```python
from build123d import *

# Parameters (mm, degrees)
PAD_DEPTH       = 15
PAD_DEPTH_BACK  = 15
SKETCH001_R     = 1.6
HOLE_DEPTH      = 25
SKETCH002_R     = 1.1
POCKET_DEPTH    = 5.801
SKETCH003_R     = 4.75
POCKET001_DEPTH = 5


with BuildPart() as part:
    # Sketch → Pad (new body, two sides)
    with BuildSketch(Plane.YZ) as pad_sk:
        Polygon((-21, 0), (-21, -5.8), (-16.2, -5.8), (-16.2, -3.3), (-15.2, -3.3), (-15.2, -1.8), (15.2, -1.8), (15.2, -3.3), (16.2, -3.3), (16.2, -5.8), (21, -5.8), (21, 0), align=None)
    extrude(amount=PAD_DEPTH)
    extrude(pad_sk.sketch, amount=-PAD_DEPTH_BACK)

    # Sketch001 → Hole (cut)
    with BuildSketch(Plane.XY):
        with Locations((-10, 17.5)):
            Circle(SKETCH001_R)
        with Locations((0, 17.5)):
            Circle(SKETCH001_R)
        with Locations((10, 17.5)):
            Circle(SKETCH001_R)
        with Locations((10, -17.5)):
            Circle(SKETCH001_R)
        with Locations((0, -17.5)):
            Circle(SKETCH001_R)
        with Locations((-10, -17.5)):
            Circle(SKETCH001_R)
    extrude(amount=-HOLE_DEPTH, mode=Mode.SUBTRACT)

    # Sketch002 → Pocket (cut, through all)
    with BuildSketch(Plane.XY):
        with Locations((-10, 10)):
            Circle(SKETCH002_R)
        with Locations((10, 10)):
            Circle(SKETCH002_R)
        with Locations((10, -10)):
            Circle(SKETCH002_R)
        with Locations((-10, -10)):
            Circle(SKETCH002_R)
    extrude(amount=-POCKET_DEPTH, mode=Mode.SUBTRACT)

    # Sketch003 → Pocket001 (cut)
    with BuildSketch(Plane.XY):
        with Locations((-8, 0)):
            Circle(SKETCH003_R)
        with Locations((8, 0)):
            Circle(SKETCH003_R)
    extrude(amount=-POCKET001_DEPTH, mode=Mode.SUBTRACT)


solid = part.part
```
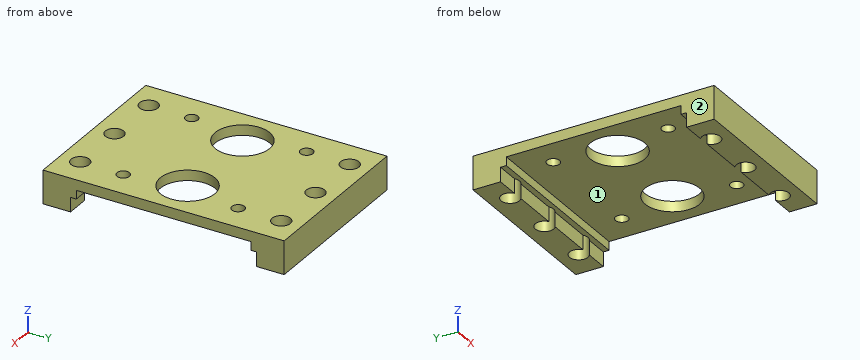
The model under review builds one solid part; all positions refer to its coordinate system, in mm. Face numbers are marked on the shaded views. A direction names the side the tool comes from. Round coordinates to 2 decimals unless told otherwise and drop trailing zeros. Write each loop counter-clockwise with the first axis right and the second up, starting at its lowest first coordinate (ties: lowest second). Pieces come first, ordered by that corner, then holes.
(1) Machinability: for the marked faces 1 and 2, which of the approach directions +Z, -Z, +X, -X, +Y, -Y give a long, thin tool a straight path to every point of the face, cutting with its end or side? Answer none if there is none.
(2) We need section B-B on y = 2.5. Give the boundary of the cut face in (x, z), and give its area (3 significant figures).
(3) We need section A-A on z = -4.25. Give the boundary of the cut face in (x, y).
(4) Insertion check: pin 1 (1 mm diameter, centred on x = -5, y = -11, fed in from -Z). The pin has a flat end and moves straight along its axis. Give the tip position at first contact, or say it passes through.
(5) We need section D-D on x = -5.5. Give the boundary of the cut face in (y, z), and give its area (3 significant figures).
(6) Wall thickness on L1, parallel to X at y = -17.5, z = -1.5; L2, parallel to Y at x = -10, z = -2.75; L3, parallel to Y at x = 0, z = -1.5: over which ranges is each line inside the solid? List them lowest first.
(7) We need section C-C on x = 10. Give the boundary of the cut face in (y, z), and give its area (3 significant figures).
Findings below:
1. face 1: -Z, +X, -X
1. face 2: +Z, -Z, -X, +Y, -Y
2. outline: (-15, -1.8) - (-12.04, -1.8) - (-12.04, 0) - (-15, 0) - close; (-3.96, -1.8) - (3.96, -1.8) - (3.96, 0) - (-3.96, 0) - close; (12.04, -1.8) - (15, -1.8) - (15, 0) - (12.04, 0) - close
2. area: 24.9 mm2
3. outline: (-15, -21) - (15, -21) - (15, -16.2) - (10.93, -16.2) arc R1.6 cw (long way) to (9.07, -16.2) - (0.93, -16.2) arc R1.6 cw (long way) to (-0.93, -16.2) - (-9.07, -16.2) arc R1.6 cw (long way) to (-10.93, -16.2) - (-15, -16.2) - close; (-15, 16.2) - (-10.93, 16.2) arc R1.6 cw (long way) to (-9.07, 16.2) - (-0.93, 16.2) arc R1.6 cw (long way) to (0.93, 16.2) - (9.07, 16.2) arc R1.6 cw (long way) to (10.93, 16.2) - (15, 16.2) - (15, 21) - (-15, 21) - close
4. pin 1: stops at z = -1.8
5. outline: (-21, -5.8) - (-16.2, -5.8) - (-16.2, -3.3) - (-15.2, -3.3) - (-15.2, -1.8) - (-4.04, -1.8) - (-4.04, 0) - (-21, 0) - close; (4.04, -1.8) - (15.2, -1.8) - (15.2, -3.3) - (16.2, -3.3) - (16.2, -5.8) - (21, -5.8) - (21, 0) - (4.04, 0) - close
5. area: 102 mm2
6. L1: x = -15 to -11.6, -8.4 to -1.6, 1.6 to 8.4, 11.6 to 15
6. L2: y = -21 to -19.1, -15.9 to -15.2, 15.2 to 15.9, 19.1 to 21
6. L3: y = -21 to -19.1, -15.9 to 15.9, 19.1 to 21
7. outline: (-21, -5.8) - (-19.1, -5.8) - (-19.1, 0) - (-21, 0) - close; (-15.9, -3.3) - (-15.2, -3.3) - (-15.2, -1.8) - (-11.1, -1.8) - (-11.1, 0) - (-15.9, 0) - close; (-8.9, -1.8) - (-4.31, -1.8) - (-4.31, 0) - (-8.9, 0) - close; (4.31, -1.8) - (8.9, -1.8) - (8.9, 0) - (4.31, 0) - close; (11.1, -1.8) - (15.2, -1.8) - (15.2, -3.3) - (15.9, -3.3) - (15.9, 0) - (11.1, 0) - close; (19.1, -5.8) - (21, -5.8) - (21, 0) - (19.1, 0) - close
7. area: 57.9 mm2
